The figure shows three views and two pictorial views of one solid part (mm, origin at its lowest corner). Answer the questions. A direction names the side the tool comes from. Give positions to 0.01 mm unless a question says otherwise; leave off trailing zeros. Write each loop counter-clockwise with the first axis right and the second up, starting at its lowest first coordinate (ties: lowest second). Pieces come first, ordered by that corner, then holes. Notation, with made-up numbers: (0.5, -38.75) -> (56.5, -38.75) arc R18 ccw to (56.5, -26.75) -> close; hole circle Ø6 at (17, 76). An arc over 180 degrees is marked (long way). Write each question's results on one line, items separated by ' | '. Start each with the question number.
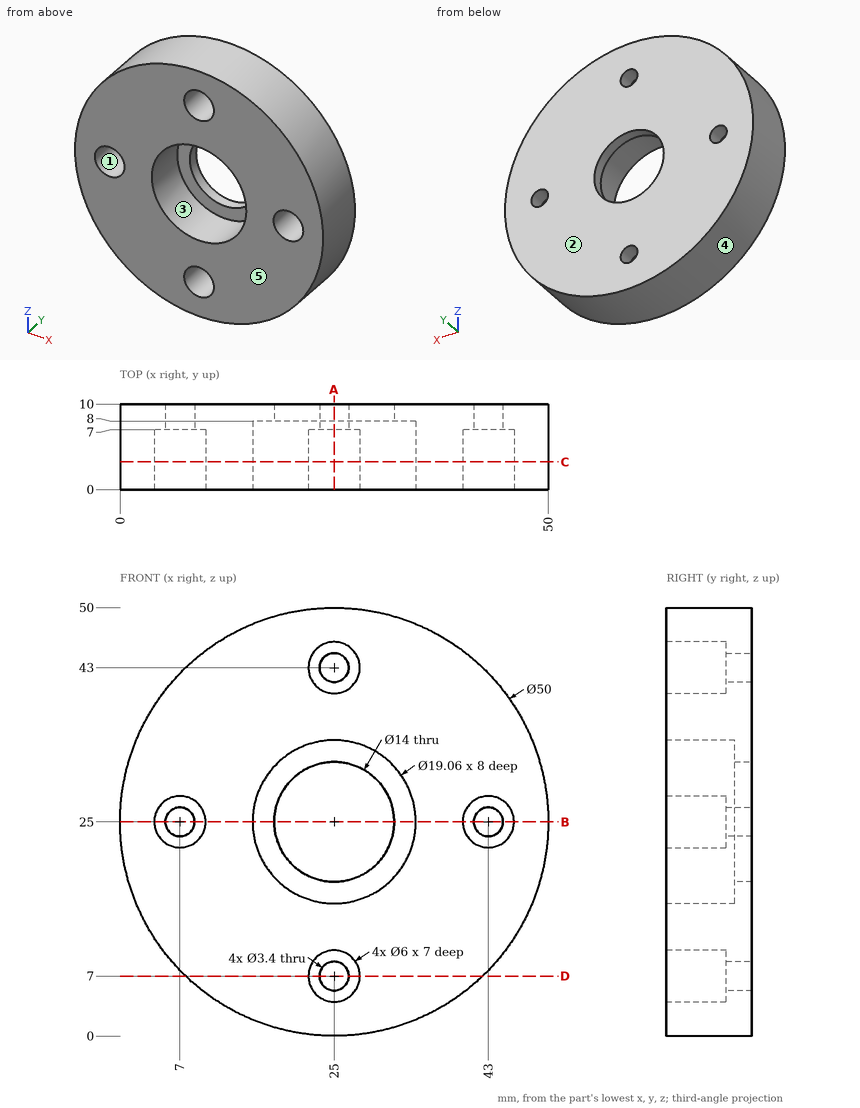
1. A tool of negligible diameter and unlimited length cuts with its end or side. For the marked faces 1 and 2, from which of +Z, -Z, +X, -X, +Y, -Y can it reach the whole face along a straight path? Write none if from no direction.
2. Section A-A (x = 25) is taken. Write down the section's boundary in (y, z).
3. Each of these flat-tipped pins is pushed along its axis until it touches: pin 1 Ø5 at (x, z) = (44, 8) entering from +Y; pin 2 Ø5.5 at (x, z) = (7, 25) entering from -Y; pin 3 Ø3 at (x, z) = (43, 25) entering from -Y; pin 4 Ø6 at (x, y) = (38, 2) entering from -Z. Where does it stop, or does it pass through?
4. Consider probe 1 along X at (y, z) = (9.15, 25); probe 2 along X at (y, z) = (4.25, 25); probe 3 along X at (y, z) = (4.5, 17). Determine where each line is inside the solid, lowest interval first. Write a range as [from, to].
5. Section D-D (z = 7) is taken. Write down the section's boundary in (x, y).
6. Section C-C (y = 3.25) is taken. Write down the section's boundary in (x, z), then the cut area to 3 significant figures.
7. The mould has two halves that part along Z. Classify the marked faces 3, 4 and 5: pulls with the +Z half, pulls with the -Z half, needs draft (parallel to the pull), parting line crosses it, or undercut.
8. Section B-B (z = 25) is taken. Write down the section's boundary in (x, y), then the cut area to 3 significant figures.
Results:
1) face 1: -Y | face 2: +Z, -Z, +X, -X, +Y
2) outline: (0, 0) -> (10, 0) -> (10, 5.3) -> (7, 5.3) -> (7, 4) -> (0, 4) -> close; (0, 10) -> (7, 10) -> (7, 8.7) -> (10, 8.7) -> (10, 18) -> (8, 18) -> (8, 15.47) -> (0, 15.47) -> close; (0, 34.53) -> (8, 34.53) -> (8, 32) -> (10, 32) -> (10, 41.3) -> (7, 41.3) -> (7, 40) -> (0, 40) -> close; (0, 46) -> (7, 46) -> (7, 44.7) -> (10, 44.7) -> (10, 50) -> (0, 50) -> close
3) pin 1: stops at y = 10 | pin 2: stops at y = 7 | pin 3: passes through | pin 4: stops at z = 2.09
4) probe 1: x = [0, 5.3], [8.7, 18], [32, 41.3], [44.7, 50] | probe 2: x = [0, 4], [10, 15.47], [34.53, 40], [46, 50] | probe 3: x = [1.31, 19.82], [30.18, 48.69]
5) outline: (7.65, 0) -> (22, 0) -> (22, 7) -> (23.3, 7) -> (23.3, 10) -> (7.65, 10) -> close; (26.7, 7) -> (28, 7) -> (28, 0) -> (42.35, 0) -> (42.35, 10) -> (26.7, 10) -> close
6) outline: circle Ø50 at (25, 25); hole circle Ø6 at (7, 25); hole circle Ø19.06 at (25, 25); hole circle Ø6 at (25, 7); hole circle Ø6 at (25, 43); hole circle Ø6 at (43, 25) | area: 1,570 mm²
7) face 3: undercut | face 4: parting line crosses it | face 5: needs draft
8) outline: (0, 0) -> (4, 0) -> (4, 7) -> (5.3, 7) -> (5.3, 10) -> (0, 10) -> close; (8.7, 7) -> (10, 7) -> (10, 0) -> (15.47, 0) -> (15.47, 8) -> (18, 8) -> (18, 10) -> (8.7, 10) -> close; (32, 8) -> (34.53, 8) -> (34.53, 0) -> (40, 0) -> (40, 7) -> (41.3, 7) -> (41.3, 10) -> (32, 10) -> close; (44.7, 7) -> (46, 7) -> (46, 0) -> (50, 0) -> (50, 10) -> (44.7, 10) -> close | area: 215 mm²
